The model under review builds one solid part; all positions refer to its coordinate system, in mm. Give positions to 0.01 mm unless a question says otherwise; leave off trailing zeros. Loops run counter-clockwise (first coordinate to the right, second up) from the corner with the lowest first, then second, coordinate; pieces in that order, holes last. Notation, with made-up numbers: (-11, 21.25) - (-4, 21.25) arc R16 cw to (-4, 32.25) - close; hole circle Ø4 at (-24, -4.75). An arc over 180 degrees is marked (long way). Answer as a JSON object with one key per item and string values.
from build123d import *

# Parameters (mm, degrees)
F0_R     = 100
F0_R_2   = 6
F0_R_3   = 9
F0_R_4   = 44.45
F1_DEPTH = 12


with BuildPart() as f1:
    # F0 (on Front) → F1 (new body)
    with BuildSketch(Plane.XZ):
        Circle(F0_R)
        with Locations((-56.568542, -56.568542)):
            Circle(F0_R_2, mode=Mode.SUBTRACT)
        with Locations((0, -80)):
            Circle(F0_R_3, mode=Mode.SUBTRACT)
        with Locations((56.568542, -56.568542)):
            Circle(F0_R_2, mode=Mode.SUBTRACT)
        with Locations((-80, 0)):
            Circle(F0_R_3, mode=Mode.SUBTRACT)
        with Locations((-56.568542, 56.568542)):
            Circle(F0_R_2, mode=Mode.SUBTRACT)
        Circle(F0_R_4, mode=Mode.SUBTRACT)
        with Locations((80, 0)):
            Circle(F0_R_3, mode=Mode.SUBTRACT)
        with Locations((0, 80)):
            Circle(F0_R_3, mode=Mode.SUBTRACT)
        with Locations((56.568542, 56.568542)):
            Circle(F0_R_2, mode=Mode.SUBTRACT)
    extrude(amount=F1_DEPTH)


solid = f1.part
Q1. Consider section C-C, the plane z = 0. State the section outline as (x, y) points, plus the area to 3 significant figures.
Results:
{"outline": "(-100, -12) - (-89, -12) - (-89, 0) - (-100, 0) - close; (-71, -12) - (-44.45, -12) - (-44.45, 0) - (-71, 0) - close; (44.45, -12) - (71, -12) - (71, 0) - (44.45, 0) - close; (89, -12) - (100, -12) - (100, 0) - (89, 0) - close", "area": "901 mm^2"}
Q2. The part is to be moulded in two halves that separate along X. For faces 1 (the face through (-1, 0, 46)), 2 (the face through (88.584, -5.916, 2.703)), 3 (the face through (95.38, -5.92, 30.04)), say which applies: +X half, -X half, draft (parallel to the pull), parting line (faces both ways), or undercut.
Results:
{"face 1": "draft", "face 2": "undercut", "face 3": "parting line"}
Q3. Consider section B-B, the plane x = 80. State the section outline as (y, z) points.
Results:
{"outline": "(-12, -60) - (0, -60) - (0, -9) - (-12, -9) - close; (-12, 9) - (0, 9) - (0, 60) - (-12, 60) - close"}
Q4. Consider section A-A, the plane z = 80. State the section outline as (x, y) points, plus the area to 3 significant figures.
Results:
{"outline": "(-60, -12) - (-9, -12) - (-9, 0) - (-60, 0) - close; (9, -12) - (60, -12) - (60, 0) - (9, 0) - close", "area": "1,220 mm^2"}
Q5. Consider section D-D, the plane x = 0. State the section outline as (y, z) points.
Results:
{"outline": "(-12, -100) - (0, -100) - (0, -89) - (-12, -89) - close; (-12, -71) - (0, -71) - (0, -44.45) - (-12, -44.45) - close; (-12, 44.45) - (0, 44.45) - (0, 71) - (-12, 71) - close; (-12, 89) - (0, 89) - (0, 100) - (-12, 100) - close"}
Q6. To check wall thickness, follow probe 1 along Z at (x, y) = (0, -9); probe 2 along X at (y, z) = (-2.25, -0.5); probe 3 along Z at (x, y) = (6, -2.75). State the ranges of each line that lie inside material, in increasing order. Write a range as [from, to].
Results:
{"probe 1": "z = [-100, -89], [-71, -44.45], [44.45, 71], [89, 100]", "probe 2": "x = [-100, -88.99], [-71.01, -44.45], [44.45, 71.01], [88.99, 100]", "probe 3": "z = [-99.82, -86.71], [-73.29, -44.04], [44.04, 73.29], [86.71, 99.82]"}
Q7. Clearance check with flat-ended pins moving along their axes: pin 1 Ø14.5 at (x, z) = (-80, 0) entering from -Y; pin 2 Ø1.5 at (y, z) = (-2.5, -38) entering from -X; pin 3 Ø6 at (x, y) = (7.5, -10.5) entering from +Z; pin 4 Ø2 at (x, y) = (41, -10.5) entering from +Z. State where each tip first meets the part, or that it passes through.
Results:
{"pin 1": "passes through", "pin 2": "stops at x = -92.8", "pin 3": "stops at z = 99.9", "pin 4": "stops at z = 91.65"}
